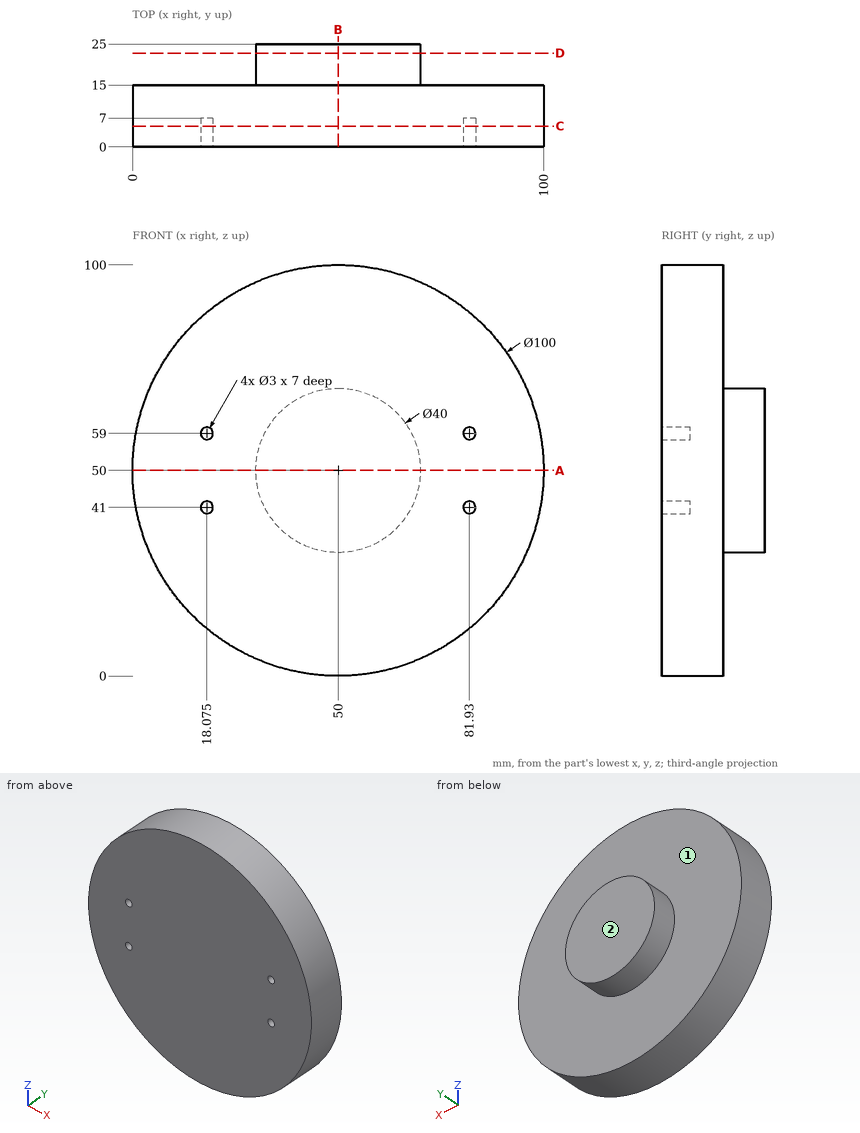
Design review of the part shown in the three views and the two pictorial views. Dimensions are in mm from the part's minimum x, y and z. A direction names the side the tool comes from. Give positions to 0.01 mm unless a question says otherwise; leave off trailing zeros. Write each loop counter-clockwise with the first axis right and the second up, starting at its lowest first coordinate (ties: lowest second). Pieces come first, ordered by that corner, then holes. Notation, with made-up numbers: M 66.25,74.5 L 100.25,74.5 A10 cw 100.25,80.5 Z; hole C -19,69.25 d2. An arc over 180 degrees is marked long. One line per question, with ' | ' between items. Start each with the question number.
Item 1: For the marked faces 1 and 2, list the 3-axis set-ups (+Z, -Z, +X, -X, +Y, -Y) from which the entire face can be reached by the end or side of a thin tool; tool diameter is ignored.
Item 2: Wall thickness on line 1 (X direction, y = 2, z = 41) (3 decimals); line 2 (Z direction, x = 81.93, y = 4.75); line 3 (Y direction, x = 20, z = 64.5): over which ranges is each line inside the solid? List them lowest first. Write a range as from..to.
Item 3: We need section B-B on x = 50. Write out the cut boundary in (y, z).
Item 4: We need section D-D on y = 22.75. Write out the cut boundary in (x, z).
Item 5: We need section C-C on y = 5. Write out the cut boundary in (x, z) (3 decimals).
Item 6: We need section A-A on z = 50. Write out the cut boundary in (x, y).
Item 7: For pin 1 (2.5 mm diameter, centred on x = 18.5, z = 59, fed in from -Y); pin 2 (1 mm diameter, centred on y = 2.5, z = 69, fed in from +X); pin 3 (4 mm diameter, centred on y = 13.5, z = 59.5, fed in from +X); pin 4 (4 mm diameter, centred on x = 81.93, z = 59, fed in from +Y), all flat-tipped, find the tip position at first contact; note any pin that passes through.
Results found:
1) face 1: +Y | face 2: +Z, -Z, +X, -X, +Y
2) line 1: x = 0.817..16.575, 19.575..80.43, 83.43..99.183 | line 2: z = 11.52..39.5, 42.5..57.5, 60.5..88.48 | line 3: y = 0..15
3) outline: M 0,0 L 15,0 L 15,30 L 25,30 L 25,70 L 15,70 L 15,100 L 0,100 Z
4) outline: C 50,50 d40
5) outline: C 50,50 d100; hole C 18.075,41 d3; hole C 18.075,59 d3; hole C 81.93,41 d3; hole C 81.93,59 d3
6) outline: M 0,0 L 100,0 L 100,15 L 70,15 L 70,25 L 30,25 L 30,15 L 0,15 Z
7) pin 1: stops at y = 0 | pin 2: stops at x = 96.45 | pin 3: stops at x = 99.43 | pin 4: stops at y = 15
